```python
from build123d import *

# Parameters (mm, degrees)
SKETCH1_W           = 82
SKETCH1_H           = 25
BOSS_EXTRUDE1_DEPTH = 12.7
SKETCH2_W           = 9.53
SKETCH2_H           = 6.2
CUT_EXTRUDE1_DEPTH  = 26
SKETCH3_R           = 4.5
CUT_EXTRUDE2_DEPTH  = 13


with BuildPart() as part:
    # Sketch1 → Boss-Extrude1 (new body)
    with BuildSketch(Plane(origin=(0, 0, 0), x_dir=(1, 0, 0), z_dir=(0, 1, 0))):
        with Locations((41, 12.5)):
            Rectangle(SKETCH1_W, SKETCH1_H)
    extrude(amount=BOSS_EXTRUDE1_DEPTH)

    # Sketch2 → Cut-Extrude1 (cut, through all)
    with BuildSketch(Plane.XY):
        with Locations((10.14, 3.1)):
            Rectangle(SKETCH2_W, SKETCH2_H)
    cut_extrude1 = extrude(amount=-CUT_EXTRUDE1_DEPTH, mode=Mode.SUBTRACT)

    # Sketch3 → Cut-Extrude2 (cut)
    with BuildSketch(Plane.XY):
        with Locations((23, 6.35)):
            Circle(SKETCH3_R)
    cut_extrude2 = extrude(amount=-CUT_EXTRUDE2_DEPTH, mode=Mode.SUBTRACT)

    # Mirror1: Cut-Extrude1, Cut-Extrude2 across plane
    add(cut_extrude1.mirror(Plane(origin=(41, 0, 0), x_dir=(0, 0, 1), z_dir=(1, 0, 0))), mode=Mode.SUBTRACT)
    add(cut_extrude2.mirror(Plane(origin=(41, 0, 0), x_dir=(0, 0, 1), z_dir=(1, 0, 0))), mode=Mode.SUBTRACT)


solid = part.part
```
For this review, take the finished solid that the model builds, in its own axes (mm). A direction names the side the tool comes from. Coordinates: 2 decimals unless noted, no trailing zeros. Order: outer loops, then holes, each group sorted by start corner. A loop starts at its lowest first (then second) coordinate and runs counter-clockwise, first axis right, second up. Notation, with made-up numbers: (66, 15.5) - (118, 15.5) arc R33 ccw to (118, 48.5) - close; hole circle Ø7 at (33.5, 45). An arc over 180 degrees is marked (long way). Answer as a JSON object with one key per item and string values. Group by question number.
1. We need section D-D on y = 4.5. State the section outline as (x, z) points (3 decimals).
2. For probe 1 along X at (y, z) = (1.25, -16.75) (3 decimals); probe 2 along Y at (x, z) = (23, -5); probe 3 along X at (y, z) = (2.25, -5.75) (3 decimals), list the stretches that pass through material, from the lowest coordinate up.
3. The part is to be moulded in two halves that separate along Y. For faces 4 (the flat face through (41, 0, -13)), 5 (the flat face through (40, 12.7, -13)), 6 (the cylindrical face through (54.708, 7.702, -6.409)), say which applies: pulls with the +Y half, pulls with the -Y half, needs draft (parallel to the pull), parting line crosses it, or undercut.
4. For faces 1 (the flat face through (59, 6, -13)), 2 (the flat face through (67.095, 3, -12)), 3 (the flat face through (3, 0, -13)), list the 3-axis set-ups (+Z, -Z, +X, -X, +Y, -Y) from which the entire face can be reached by the end or side of a thin tool; tool diameter is ignored.
5. We need section A-A on z = -3. State the section outline as (x, y) points (3 decimals), then the cut area to 3 significant figures.
6. We need section B-B on x = 59. State the section outline as (y, z) points, then the cut area to 4 significant figures.
7. We need section C-C on z = -15. State the section outline as (x, y) points (3 decimals), then the cut area to 3 significant figures.
8. Clearance check with flat-ended pins moving along their axes: P1, Ø4.5, axis at x = 22, y = 5, coming from the +Z side; P2, Ø5, axis at x = 10.5, z = -16.5, coming from the -Y side. State where each tip first meets the part, or that it passes through.
Final values:
{
 "1": {"outline": "(0, -25) - (5.375, -25) - (5.375, 0) - (0, 0) - close; (14.905, -25) - (67.095, -25) - (67.095, 0) - (63.102, 0) - (63.102, -13) - (54.898, -13) - (54.898, 0) - (27.102, 0) - (27.102, -13) - (18.898, -13) - (18.898, 0) - (14.905, 0) - close; (76.625, -25) - (82, -25) - (82, 0) - (76.625, 0) - close"},
 "2": {"probe 1": "0 to 5.375, 14.905 to 67.095, 76.625 to 82", "probe 2": "0 to 1.85, 10.85 to 12.7", "probe 3": "0 to 5.375, 14.905 to 21.145, 24.855 to 57.145, 60.855 to 67.095, 76.625 to 82"},
 "3": {"face 4": "pulls with the -Y half", "face 5": "pulls with the +Y half", "face 6": "undercut"},
 "4": {"face 1": "+Z", "face 2": "+Z, -Z, -Y", "face 3": "+Z, -Z, +X, -X, -Y"},
 "5": {"outline": "(0, 0) - (5.375, 0) - (5.375, 6.2) - (14.905, 6.2) - (14.905, 0) - (67.095, 0) - (67.095, 6.2) - (76.625, 6.2) - (76.625, 0) - (82, 0) - (82, 12.7) - (0, 12.7) - close; hole circle Ø9 at (23, 6.35); hole circle Ø9 at (59, 6.35)", "area": "796 mm²"},
 "6": {"outline": "(0, -25) - (12.7, -25) - (12.7, 0) - (10.85, 0) - (10.85, -13) - (1.85, -13) - (1.85, 0) - (0, 0) - close", "area": "200.5 mm²"},
 "7": {"outline": "(0, 0) - (5.375, 0) - (5.375, 6.2) - (14.905, 6.2) - (14.905, 0) - (67.095, 0) - (67.095, 6.2) - (76.625, 6.2) - (76.625, 0) - (82, 0) - (82, 12.7) - (0, 12.7) - close", "area": "923 mm²"},
 "8": {"P1": "z = -13", "P2": "y = 6.2"}
}
